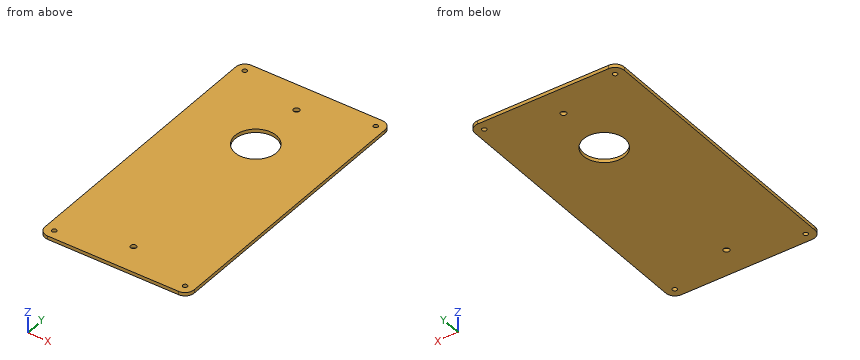
Autodesk Fusion 360 part; units mm, degrees
sketch "Sketch1" plane through (0, 0, 0) normal (0, 0, 1) x (1, 0, 0)
  line L0 (65, 125) -> (-65, 125)
  line L1 (-65, 125) -> (-65, -125)
  line L2 (-65, -125) -> (65, -125)
  line L3 (65, -125) -> (65, 125)
  line L4 (65, 125) -> (-65, -125) construction
  line L5 (-65, 125) -> (65, -125) construction
  dimension "d1" = 130
  dimension "d2" = 250
extrude "Extrude1" add sketch "Sketch1" along normal blind 3
sketch "Sketch2" plane through (0, 0, 3) normal (0, 0, 1) x (-1, 0, 0)
  line L0 (-65, 125) -> (-65, -125)
  line L1 (-65, -125) -> (65, -125)
  line L2 (65, -125) -> (65, 125)
  line L3 (65, 125) -> (-65, 125)
  circle A0 centre (0, -50) radius 18
  circle A1 centre (0, -100) radius 2.5
  circle A2 centre (0, 100) radius 2.5
  dimension "d7" = 5
  dimension "d8" = 5
extrude "Extrude2" cut sketch "Sketch2" against normal blind 3 contours A0 | A1 | A2
fillet "Fillet1" radius 8 4 edges at (65, -125, 1.5) (-65, -125, 1.5) (-65, 125, 1.5) (65, 125, 1.5)
sketch "Sketch3" plane through (0, 0, 3) normal (0, 0, 1) x (-1, 0, 0)
  circle A0 centre (0, 100) radius 2.5
  circle A1 centre (0, -50) radius 18
  circle A2 centre (0, -100) radius 2.5
  arc A3 (-65, -117) -> (-57, -125) centre (-57, -117) ccw
  line L0 (-57, -125) -> (57, -125)
  arc A4 (57, -125) -> (65, -117) centre (57, -117) ccw
  line L1 (65, -117) -> (65, 117)
  arc A5 (65, 117) -> (57, 125) centre (57, 117) ccw
  line L2 (57, 125) -> (-57, 125)
  arc A6 (-57, 125) -> (-65, 117) centre (-57, 117) ccw
  line L3 (-65, 117) -> (-65, -117)
  circle A7 centre (-57, 117) radius 2
  circle A8 centre (57, 117) radius 2
  circle A9 centre (57, -117) radius 2
  circle A10 centre (-57, -117) radius 2
  dimension "d13" = 4
  dimension "d14" = 4
  dimension "d15" = 4
  dimension "d16" = 4
extrude "Extrude3" cut sketch "Sketch3" against normal blind 3 contours A7 | A8 | A9 | A10
Build history of the part. All positions in model axes, mm. Round coordinates to 2 decimals unless told otherwise and drop trailing zeros. Loops run counter-clockwise (first coordinate to the right, second up) from the corner with the lowest first, then second, coordinate; pieces in that order, holes last. Notation, with made-up numbers: (-25, 36.25) -> (-7, 36.25) arc R24 cw to (-7, 46.25) -> close; hole circle Ø4 at (4.5, -6). An arc over 180 degrees is marked (long way). One line per item, written item: value. Start each with the question number.
Q1. Cut at C-C on y = -100. List the corners of the cut face in (x, z).
Q2. Cut at D-D on y = 52.5. List the corners of the cut face in (x, z).
Q3. Cut at A-A on x = 0. List the corners of the cut face in (y, z), plus the area to 3 significant figures.
Q4. Probe line 1 along X through (y, z) = (117, 1.5); line 2 along Y through (x, z) = (0, 2); line 3 along X through (y, z) = (100, 0.7). List the from-to ranges inside material, lowest first.
Q5. Cut at B-B on z = 2.15. List the corners of the cut face in (x, y).
Computed:
1. outline: (-65, 0) -> (-2.5, 0) -> (-2.5, 3) -> (-65, 3) -> close; (2.5, 0) -> (65, 0) -> (65, 3) -> (2.5, 3) -> close
2. outline: (-65, 0) -> (-17.83, 0) -> (-17.83, 3) -> (-65, 3) -> close; (17.83, 0) -> (65, 0) -> (65, 3) -> (17.83, 3) -> close
3. outline: (-125, 0) -> (-102.5, 0) -> (-102.5, 3) -> (-125, 3) -> close; (-97.5, 0) -> (32, 0) -> (32, 3) -> (-97.5, 3) -> close; (68, 0) -> (97.5, 0) -> (97.5, 3) -> (68, 3) -> close; (102.5, 0) -> (125, 0) -> (125, 3) -> (102.5, 3) -> close
3. area: 612 mm²
4. line 1: -65 to -59, -55 to 55, 59 to 65
4. line 2: -125 to -102.5, -97.5 to 32, 68 to 97.5, 102.5 to 125
4. line 3: -65 to -2.5, 2.5 to 65
5. outline: (-65, -117) arc R8 ccw to (-57, -125) -> (57, -125) arc R8 ccw to (65, -117) -> (65, 117) arc R8 ccw to (57, 125) -> (-57, 125) arc R8 ccw to (-65, 117) -> close; hole circle Ø4 at (-57, -117); hole circle Ø4 at (-57, 117); hole circle Ø36 at (0, 50); hole circle Ø5 at (0, -100); hole circle Ø5 at (0, 100); hole circle Ø4 at (57, -117); hole circle Ø4 at (57, 117)
